Geometry check sheet. Reference: drawing and pictorial views, mm from the part's lowest x, y, z. A direction names the side the tool comes from. Give positions to 0.01 mm unless a question says otherwise; leave off trailing zeros. Loops run counter-clockwise (first coordinate to the right, second up) from the corner with the lowest first, then second, coordinate; pieces in that order, holes last. Notation, with made-up numbers: (11.25, 45) -> (70.25, 45) arc R12 ccw to (70.25, 61) -> close; hole circle Ø6 at (18.5, 71). An arc over 180 degrees is marked (long way). One line per item, written item: value. Start each with the question number.
(1) Scan lines: line 1 along X through (y, z) = (3, 23.25); line 2 along Z through (x, y) = (2, 5); line 3 along Y through (x, z) = (1.75, 19.5) (1 decimal). Record each from-to range of solid material in increasing order. Write a range as from..to.
(2) Gauge pin test, flat end, axial feed: pin 1 Ø3 at (y, z) = (2.5, 3.5) entering from -X. Record the tip position at first contact, or that the pin passes through.
(3) Tool access check on the marked faces 1 and 2. Record the directions out of +Z, -Z, +X, -X, +Y, -Y that give a thin tool (end or side, any length) a straight path to the whole face; none if there is none.
(4) Sectioned sample at B-B, the plane z = 4.5. Record the cut outline in (x, y).
(5) Draft check along Y on the marked faces 3, 4, 5 and 6. Enter one of: pulls with the +Y half, pulls with the -Y half, needs draft (parallel to the pull), parting line crosses it, or undercut.
(6) Sectioned sample at A-A, the plane z = 17.5. Record the cut outline in (x, y) (1 decimal).
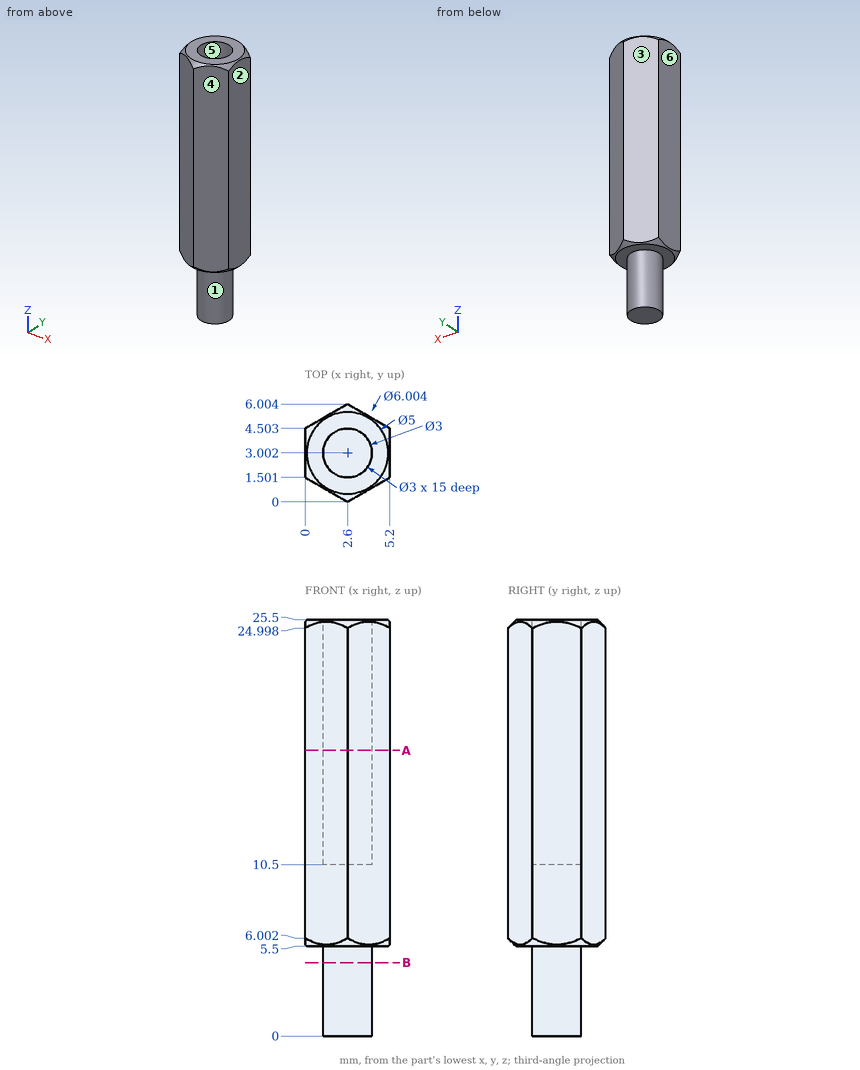
Calculated:
1. line 1: x = 0..1.1, 4.1..5.2
1. line 2: z = 5.5..25.5
1. line 3: y = 0.5..1.8, 4.2..5.5
2. pin 1: stops at x = 1.1
3. face 1: -Z
3. face 2: +Z, -Z, +X, +Y, -Y
4. outline: circle Ø3 at (2.6, 3)
5. face 3: pulls with the +Y half
5. face 4: pulls with the -Y half
5. face 5: undercut
5. face 6: needs draft
6. outline: (0, 1.5) -> (2.6, 0) -> (5.2, 1.5) -> (5.2, 4.5) -> (2.6, 6) -> (0, 4.5) -> close; hole circle Ø3 at (2.6, 3)
